```python
from build123d import *

# Parameters (mm, degrees)
F0_W      = 85
F0_H      = 150
F0_R      = 2
F1_DEPTH  = 158
F2_R      = 2
F3_DEPTH  = 15
F4_W      = 12
F4_H      = 18
F4_W_2    = 22
F4_H_2    = 30
F5_DEPTH  = 5.58503
F6_W      = 17.8319794536
F6_H      = 25.8319794536
F7_DEPTH  = 9.40301
F8_R      = 50.7166992879
F9_DEPTH  = 3
F10_W     = 36.3819319755
F10_H     = 12.9120806232
F11_DEPTH = 22.01429
F12_W     = 36.3819319755
F12_H     = 15.4613213601
F13_DEPTH = 105.26626


with BuildPart() as f1:
    # F0 (on Front) → F1 (new body)
    with BuildSketch(Plane.XZ):
        with Locations((42.5, 75)):
            Rectangle(F0_W, F0_H)
        with Locations((5, 30)):
            Circle(F0_R, mode=Mode.SUBTRACT)
        with Locations((79, 6.5)):
            Circle(F0_R, mode=Mode.SUBTRACT)
        with Locations((15.5, 143.5)):
            Circle(F0_R, mode=Mode.SUBTRACT)
        with Locations((79, 143.5)):
            Circle(F0_R, mode=Mode.SUBTRACT)
        with Locations((15.5, 143.5)):
            Circle(F0_R)
        with Locations((79, 143.5)):
            Circle(F0_R)
        with Locations((79, 6.5)):
            Circle(F0_R)
        with Locations((5, 30)):
            Circle(F0_R)
    extrude(amount=F1_DEPTH)

    # F2 (on face) → F3 (cut)
    with BuildSketch(Plane.XZ.offset(158)):
        with Locations((79, 6.5)):
            Circle(F2_R)
        with Locations((5, 30)):
            Circle(F2_R)
        with Locations((15.5, 143.5)):
            Circle(F2_R)
        with Locations((79, 143.5)):
            Circle(F2_R)
    extrude(amount=-F3_DEPTH, mode=Mode.SUBTRACT)

    # F4 (on face) → F5 (join)
    with BuildSketch(Plane.XZ.offset(158)):
        with Locations((22, 32)):
            Rectangle(F4_W, F4_H)
        with Locations((47, 32)):
            Rectangle(F4_W_2, F4_H_2)
    extrude(amount=F5_DEPTH)

    # F6 (on face) → F7 (cut)
    with BuildSketch(Plane.XZ.offset(163.58503)):
        with Locations((47, 32)):
            Rectangle(F6_W, F6_H)
    extrude(amount=-F7_DEPTH, mode=Mode.SUBTRACT)

    # F8 (on face) → F9 (join)
    with BuildSketch(Plane.YZ.offset(85)):
        with Locations((-82.3336839676, 69.8694512248)):
            Circle(F8_R)
    extrude(amount=F9_DEPTH)

    # F10 (on face) → F11 (join)
    with BuildSketch(Plane.XZ):
        with Locations((35.7437124476, 14.9440853857)):
            Rectangle(F10_W, F10_H)
    extrude(amount=-F11_DEPTH)

    # F12 (on face) → F13 (join)
    with BuildSketch(Plane.XY.offset(21.4001256973)):
        with Locations((35.7437124476, 14.2836293199)):
            Rectangle(F12_W, F12_H)
    extrude(amount=F13_DEPTH)


solid = f1.part
```
Geometry check sheet. Reference: the model listing, model coordinates, mm. A direction names the side the tool comes from. Round coordinates to 2 decimals unless told otherwise and drop trailing zeros. Order: outer loops, then holes, each group sorted by start corner. A loop starts at its lowest first (then second) coordinate and runs counter-clockwise, first axis right, second up. Notation, with made-up numbers: (67, 81.25) -> (118, 81.25) arc R10 ccw to (118, 96.25) -> close; hole circle Ø3 at (-22, 82). An arc over 180 degrees is marked (long way). Return JSON: item names as keys, results as strings. Group by question number.
Q1. Section check C-C, the plane x = 70.5. Record the boundary of the cut face in (y, z).
Q2. Tool access check on faces 1 (the flat face through (35, 11, 8.488)), 2 (the flat face through (47, -154.182, 32)), 3 (the flat face through (85, -43, 107)). Record the directions out of +Z, -Z, +X, -X, +Y, -Y that give a thin tool (end or side, any length) a straight path to the whole face; none if there is none.
Q3. Section check D-D, the plane y = -9. Record the boundary of the cut face in (x, z), plus the area to 4 significant figures.
Q4. Release check for a two-part mould opening along Z. For faces 4 (the flat face through (22, -161, 23)), 5 (the flat face through (22, -161, 41)), 6 (the flat face through (47, -159, 19.084)) record: released by +Z, released by -Z, zero draft, split by the parting line, or undercut.
Q5. Gauge pin test, flat ends, axial feed: pin 1 (4.5 mm diameter, centred on x = 52.5, y = -161, fed in from -Z); pin 2 (12.5 mm diameter, centred on x = 32, y = 16, fed in from +Z); pin 3 (2 mm diameter, centred on x = 56, y = -66, fed in from -Z); pin 4 (17.5 mm diameter, centred on x = 36.5, y = 12, fed in from -Z). Record the tip position at first contact, or that the pin passes through.
Q6. Material ranges on probe 1 along Z at (x, y) = (79, -150); probe 2 along Y at (x, z) = (51.5, 59); probe 3 along Y at (x, z) = (53, 26), recorded low to high. Write a range as from..to.
Q7. Section check A-A, the plane z = 60. Record the boundary of the cut face in (x, y), plus the area to 3 significant figures.
Q8. Section check B-B, the plane z = 37. Record the boundary of the cut face in (x, y), plus the area to 3 significant figures.
Numbers:
{
 "1": {"outline": "(-158, 0) -> (0, 0) -> (0, 150) -> (-158, 150) -> close"},
 "2": {"face 1": "-Z, +X, -X, +Y", "face 2": "-Y", "face 3": "+X"},
 "3": {"outline": "(0, 0) -> (85, 0) -> (85, 150) -> (0, 150) -> close", "area": "12,750 mm^2"},
 "4": {"face 4": "released by -Z", "face 5": "released by +Z", "face 6": "undercut"},
 "5": {"pin 1": "z = 17", "pin 2": "z = 126.67", "pin 3": "z = 0", "pin 4": "z = 8.49"},
 "6": {"probe 1": "0..4.5, 8.5..141.5, 145.5..150", "probe 2": "-158..0, 6.55..22.01", "probe 3": "-154.18..0, 6.55..22.01"},
 "7": {"outline": "(0, -158) -> (85, -158) -> (85, -132.08) -> (88, -132.08) -> (88, -32.59) -> (85, -32.59) -> (85, 0) -> (0, 0) -> close; (17.55, 6.55) -> (53.93, 6.55) -> (53.93, 22.01) -> (17.55, 22.01) -> close", "area": "14,300 mm^2"},
 "8": {"outline": "(0, -158) -> (16, -158) -> (16, -163.59) -> (28, -163.59) -> (28, -158) -> (36, -158) -> (36, -163.59) -> (38.08, -163.59) -> (38.08, -154.18) -> (55.92, -154.18) -> (55.92, -163.59) -> (58, -163.59) -> (58, -158) -> (85, -158) -> (85, -120.96) -> (88, -120.96) -> (88, -43.71) -> (85, -43.71) -> (85, 0) -> (0, 0) -> close; (17.55, 6.55) -> (53.93, 6.55) -> (53.93, 22.01) -> (17.55, 22.01) -> close", "area": "14,200 mm^2"}
}
